Design review of the part built by this model. Coordinates are the model's own, in mm. A direction names the side the tool comes from. Coordinates: 2 decimals unless noted, no trailing zeros. Write each loop counter-clockwise with the first axis right and the second up, starting at its lowest first coordinate (ties: lowest second). Pieces come first, ordered by that corner, then holes. Notation, with made-up numbers: M 72,34 L 115,34 A14 cw 115,45 Z; hole C -2.75,40 d8. An arc over 180 degrees is marked long. One line per question, with ' | ' between items.
from build123d import *

# Parameters (mm, degrees)
F0_W           = 323.85
F0_H           = 203.2
F1_DEPTH       = 9.525
F2_R           = 2.54
F4_D           = 2.7178
F4_CSINK_D     = 2.9718
F4_CSINK_ANGLE = 82
F5_W           = 101.6
F5_H           = 35.052
F6_DEPTH       = 25.4
F7_R           = 5.08
F10_D          = 19.05
F11_DEPTH      = 25.4


with BuildPart() as f1:
    # F0 (on Top) → F1 (new body)
    with BuildSketch(Plane.XY):
        with Locations((-161.925, 101.6)):
            Rectangle(F0_W, F0_H)
    extrude(amount=F1_DEPTH)

    # F2
    f2_edges = [f1.edges().sort_by_distance(p)[0] for p in [
        (0, 0, 4.7625),
        (0, 203.2, 4.7625),
        (-323.85, 203.2, 4.7625),
        (-323.85, 0, 4.7625),
    ]]
    fillet(f2_edges, radius=F2_R)

    # F4 (through all)
    with Locations(Plane.XY.offset(9.525)):
        with Locations((-280.9748, 157.734), (-233.3498, 157.734), (-233.3498, 86.868), (-280.9748, 86.868), (-280.9748, 32.766), (-233.3498, 32.766), (-183.896, 193.04), (-158.496, 193.04), (-133.096, 193.04), (-107.696, 193.04), (-107.696, 162.306), (-133.096, 162.306), (-158.496, 162.306), (-183.896, 162.306), (-95.25, 154.432), (-95.25, 122.682), (-69.858725, 155.0977), (-69.85, 123.3477), (-38.108725, 154.432), (-38.1, 122.682001), (-12.708725, 154.432), (-12.7, 122.682)):
            CounterSinkHole(F4_D / 2, F4_CSINK_D / 2, counter_sink_angle=F4_CSINK_ANGLE)

    # F5 (on face) → F6 (cut)
    with BuildSketch(Plane.XY.offset(9.525)):
        with Locations((-250.453002, 109.474)):
            Rectangle(F5_W, F5_H)
    extrude(amount=-F6_DEPTH, mode=Mode.SUBTRACT)

    # F7
    f7_edges = [f1.edges().sort_by_distance(p)[0] for p in [
        (-301.253002, 91.948, 4.7625),
        (-301.253002, 127, 4.7625),
        (-199.653002, 127, 4.7625),
        (-199.653002, 91.948, 4.7625),
    ]]
    fillet(f7_edges, radius=F7_R)

    # F10 (through all)
    with Locations(Plane.XY.offset(9.525)):
        with Locations((-29.697825, 46.492874)):
            Hole(F10_D / 2)

    # F8 (on face) → F11 (cut)
    with BuildSketch(Plane.XY.offset(9.525)):
        with BuildLine():
            Line((-190.5, 0), (-2.54, 0))
            ThreePointArc((-2.54, 0), (-0.743949, 0.743949), (0, 2.54))
            Line((0, 2.54), (0, 88.9))
            Line((0, 88.9), (-139.7, 88.9))
            ThreePointArc((-139.7, 88.9), (-175.621024, 74.021024), (-190.5, 38.1))
            Line((-190.5, 38.1), (-190.5, 0))
        make_face()
    extrude(amount=-F11_DEPTH, mode=Mode.SUBTRACT)


solid = f1.part
1. Take a section at A-A (x = -218). Write out the cut boundary in (y, z) (3 decimals).
Answer sheet:
outline: M 0,0 L 91.948,0 L 91.948,9.525 L 0,9.525 Z; M 127,0 L 203.2,0 L 203.2,9.525 L 127,9.525 Z
2. To check wall thickness, follow line 1 along Y through (x, z) = (-38.5, 3.5); line 2 along Y through (x, z) = (-12.7, 2); line 3 along X through (y, z) = (105, 5.75). State the ranges of each line that lie inside material, in increasing order. Write a range as [from, to].
Answer sheet:
line 1: [88.9, 121.38], [123.98, 153.13], [155.73, 203.2] | line 2: [88.9, 121.32], [124.04, 153.07], [155.79, 203.2] | line 3: [-323.85, -301.25], [-199.65, 0]
3. Take a section at D-D (z = 1.75). Count the separate pieces of the cut face and the enclosed holes in it, then the cut area to 3 significant figures.
Answer sheet:
separate pieces: 1 | enclosed holes: 23 | area: 45,800 mm^2
4. Tool access review of faces 1 (the face through (-251, 127, 5)), 2 (the face through (-190.5, 19, 5)), 3 (the face through (-323.85, 100, 5)): name each direction out of +Z, -Z, +X, -X, +Y, -Y from which nothing blocks a thin tool from reaching the whole face with its end or side.
Answer sheet:
face 1: +Z, -Z | face 2: +Z, -Z, +X, -Y | face 3: +Z, -Z, -X, +Y, -Y
5. Draft analysis for pull direction Y (two halves, no side actions). For faces 4 (the face through (-199.653, 109, 5)), 5 (the face through (-69, 88.9, 5)), 6 (the face through (-200, 126, 9.525)), state which applies: pulls with the +Y half, pulls with the -Y half, needs draft (parallel to the pull), parting line crosses it, or undercut.
Answer sheet:
face 4: undercut | face 5: pulls with the -Y half | face 6: needs draft
6. Take a section at C-C (x = -74.5). Write out the cut boundary in (y, z) (3 decimals), then the cut area to 3 significant figures.
Answer sheet:
outline: M 88.9,0 L 203.2,0 L 203.2,9.525 L 88.9,9.525 Z | area: 1,090 mm^2
7. Take a section at B-B (y = 25.5). Write out the cut boundary in (x, z) (3 decimals).
Answer sheet:
outline: M -323.85,0 L -190.5,0 L -190.5,9.525 L -323.85,9.525 Z
8. Insertion check: pin 1 Ø2 at (x, y) = (-233.35, 86.87) entering from -Z; pin 2 Ø1 at (x, z) = (-59.5, 6.5) entering from -Y; pin 3 Ø5 at (x, z) = (-175.5, 7) entering from -Y; pin 4 Ø3 at (x, z) = (-149.5, 4) entering from -Y. Each pin has a flat end and moves straight along its axis. Give the tip position at first contact, or say it passes through.
Answer sheet:
pin 1: through | pin 2: y = 88.9 | pin 3: y = 71.47 | pin 4: y = 87.63
